from build123d import *
from build123d.topology import SkipClean

# Parameters (mm, degrees)
SKETCH1_R           = 1.323033288
SKETCH1_W           = 3.194492506
SKETCH1_H           = 3.000146449
SKETCH1_W_2         = 3.194434014
SKETCH1_H_2         = 6.000288014
SKETCH1_H_3         = 6.000224533
SKETCH1_W_3         = 4.990971694
SKETCH1_H_4         = 3.200091917
SKETCH1_W_4         = 4.991186163
SKETCH1_W_5         = 22.959409558
SKETCH1_H_5         = 12.40053533
BOSS_EXTRUDE1_DEPTH = 3.175


with BuildPart() as part:
    # Sketch1 → Boss-Extrude1 (new body)
    with SkipClean():  # the faces are left unmerged after this step: merging them gives an invalid solid
        with BuildSketch(Plane(origin=(0, 0, 0), x_dir=(1, 0, 0), z_dir=(0, 1, 0))):
            with BuildLine():
                Line((25.442900716, -27.532431428), (-28.456084878, -27.532431428))
                ThreePointArc((-28.456084878, -27.532431428), (-30.577373887, -26.653764751), (-31.456040564, -24.532475742))
                Line((-31.456040564, -24.532475742), (-31.456040564, 13.269326446))
                ThreePointArc((-31.456040564, 13.269326446), (-31.352979308, 14.049412081), (-31.050867612, 14.775968165))
                Line((-31.050867612, 14.775968165), (-26.174789125, 23.186205164))
                ThreePointArc((-26.174789125, 23.186205164), (-24.390968499, 24.809261571), (-21.997773241, 25.107497345))
                Line((-21.997773241, 25.107497345), (25.983223234, 16.219991273))
                ThreePointArc((25.983223234, 16.219991273), (27.743957441, 15.188191581), (28.437804204, 13.268980227))
                Line((28.437804204, 13.268980227), (28.437609204, -24.537738386))
                ThreePointArc((28.437609204, -24.537738386), (27.560473935, -26.65530708), (25.442900716, -27.532431428))
            make_face()
            with Locations(Location((-22.724218332, 21.185636807, 0), (0, 0, 270))):
                Circle(SKETCH1_R, mode=Mode.SUBTRACT)
            with Locations(Location((-26.963965218, -16.232064957, 0), (0, 0, 270))):
                Circle(SKETCH1_R, mode=Mode.SUBTRACT)
            with Locations(Location((7.974006473, 13.76898446, 0), (0, 0, 270))):
                Circle(SKETCH1_R, mode=Mode.SUBTRACT)
            with Locations(Location((7.974006472, -6.031549942, 0), (0, 0, 270))):
                Circle(SKETCH1_R, mode=Mode.SUBTRACT)
            with Locations(Location((24.045515173, -16.23206496, 0), (0, 0, 270))):
                Circle(SKETCH1_R, mode=Mode.SUBTRACT)
            Polygon((22.448181182, -10.478708085), (22.448181182, -10.484914569), (22.448181182, -12.731920553), (25.642673688, -12.731920553), (25.642673688, -10.478708085), align=None, mode=Mode.SUBTRACT)
            with Locations((24.045427435, -21.232282591)):
                Rectangle(SKETCH1_W, SKETCH1_H, mode=Mode.SUBTRACT)
            with Locations((-27.063830275, -9.731776544)):
                Rectangle(SKETCH1_W_2, SKETCH1_H_2, mode=Mode.SUBTRACT)
            with Locations((-27.063830276, -22.732321631)):
                Rectangle(SKETCH1_W_2, SKETCH1_H_3, mode=Mode.SUBTRACT)
            with Locations((18.446511119, -21.132309856)):
                Rectangle(SKETCH1_W_3, SKETCH1_H_4, mode=Mode.SUBTRACT)
            with Locations((10.460708795, -21.132309856)):
                Rectangle(SKETCH1_W_4, SKETCH1_H_4, mode=Mode.SUBTRACT)
            Polygon((-10.993335433, -19.532644781), (-10.993335433, -19.566758469), (-23.970138696, -19.566758469), (-23.970138696, -22.766982231), (-10.993335433, -22.766982231), align=None, mode=Mode.SUBTRACT)
            with Locations((7.974006472, 4.268713184)):
                Rectangle(SKETCH1_W_5, SKETCH1_H_5, mode=Mode.SUBTRACT)
            Polygon((25.642673689, -6.725489536), (25.642673689, -6.731632539), (22.448181183, -6.731632539), (22.448181183, -8.978702004), (25.642673689, -8.978702004), align=None, mode=Mode.SUBTRACT)
        extrude(amount=BOSS_EXTRUDE1_DEPTH)
    add(part.part.scale(1), mode=Mode.REPLACE)  # the faces are merged on a copy


solid = part.part
Verification items for the finished model (mm, model axes). A direction names the side the tool comes from. Coordinates: 2 decimals unless noted, no trailing zeros. Order: outer loops, then holes, each group sorted by start corner. A loop starts at its lowest first (then second) coordinate and runs counter-clockwise, first axis right, second up. Notation, with made-up numbers: M 56.25,75.25 L 111.25,75.25 A10 ccw 111.25,87.25 Z; hole C 53,70.5 d3. An arc over 180 degrees is marked long. One line per item, written item: value. Start each with the question number.
Item 1: Depth check by flat-ended pin: P1, Ø1, axis at x = -15.5, z = 19, coming from the -Y side; P2, Ø1, axis at x = -9.5, y = 0.5, coming from the -Z side. Enter the tip coordinate at first touch or a pass-through.
Item 2: Access from +Z, -Z, +X, -X, +Y, -Y to the whole of each face (thin tool, end or side, straight path). Record for faces 4 (the flat face through (12.956, 2, 21)), 5 (the flat face through (-31.456, 2, 6)).
Item 3: Sectioned sample at A-A on x = 18. Record the cut outline in (y, z) (3 decimals), then the cut area to 3 significant figures.
Item 4: Thickness scan on probe 1 along X at (y, z) = (1.15, 22.5); probe 2 along Z at (x, y) = (-25.5, 2.05); probe 3 along X at (y, z) = (0.95, -6.5). Record the ranges inside material, lowest first.
Item 5: Sectioned sample at D-D on z = -1.5. Record the cut outline in (x, y) (3 decimals), then the cut area to 3 significant figures.
Item 6: Sectioned sample at C-C on x = -1.5. Record the cut outline in (y, z) (3 decimals).
Item 7: Sectioned sample at B-B on z = 12. Record the cut outline in (x, y) (3 decimals).
Item 8: Mould release check, pull along Z, two halves, no side actions. Record for faces 1 (the flat face through (25.643, 2, 12)), 2 (the flat face through (-1, 3.175, 7)), 3 (the flat face through (1.657, 1.565, -20.726)): pulls with the +Z half, pulls with the -Z half, needs draft (parallel to the pull), parting line crosses it, or undercut.
Calculated:
1. P1: y = 0
1. P2: z = -22.89
2. face 4: +Y, -Y
2. face 5: +Z, -Z, -X, +Y, -Y
3. outline: M 0,-17.699 L 3.175,-17.699 L 3.175,-10.469 L 0,-10.469 Z; M 0,1.932 L 3.175,1.932 L 3.175,19.532 L 0,19.532 Z; M 0,22.732 L 3.175,22.732 L 3.175,27.532 L 0,27.532 Z
3. area: 94.1 mm^2
4. probe 1: -31.46 to -28.66, -25.47 to -23.97, -10.99 to 7.97, 12.96 to 15.95, 20.94 to 22.45, 25.64 to 28.44
4. probe 2: -24.05 to 6.73, 12.73 to 19.73, 25.73 to 27.53
4. probe 3: -31.46 to -3.51, 19.45 to 28.44
5. outline: M -31.456,0 L -3.506,0 L -3.506,3.175 L -31.456,3.175 Z; M 19.454,0 L 28.438,0 L 28.438,3.175 L 19.454,3.175 Z
5. area: 117 mm^2
6. outline: M 0,-21.311 L 3.175,-21.311 L 3.175,-10.469 L 0,-10.469 Z; M 0,1.932 L 3.175,1.932 L 3.175,27.532 L 0,27.532 Z
7. outline: M -31.456,0 L -28.661,0 L -28.661,3.175 L -31.456,3.175 Z; M -25.467,0 L 22.448,0 L 22.448,3.175 L -25.467,3.175 Z; M 25.643,0 L 28.438,0 L 28.438,3.175 L 25.643,3.175 Z
8. face 1: undercut
8. face 2: needs draft
8. face 3: pulls with the -Z half
